Input: part model. Units: mm. Frame: model coordinates. A direction names the side the tool comes from. Coordinates: 2 decimals unless noted, no trailing zeros. Write each loop counter-clockwise with the first axis right and the second up, starting at its lowest first coordinate (ties: lowest second). Pieces come first, ordered by that corner, then holes. Notation, with made-up numbers: (52, 28) - (71, 28) arc R17 ccw to (71, 35) - close; hole circle Ø3 at (70, 41.25). An arc over 180 degrees is marked (long way). Put each result on its own line as item: value. Start each with the question number.
1. Cut plane C-C, the plane y = 31.5. Return loops of the section in (x, z), and give its area (3 significant figures).
2. Pull-direction query (X, two-part tool) for faces 1 (the flat face through (1, 10, -42)), 2 (the flat face through (60, 10, 0)), 3 (the flat face through (-32, 10, -37)), 4 (the cylindrical face through (-60.859, 21.256, -40.797)); classes: released by +X, released by -X, zero draft, split by the parting line, or undercut.
3. Line query: line 1 (Z direction, x = 47, y = 7); line 2 (X direction, y = 10.5, z = 24.5); line 3 (Z direction, x = -31, y = 17). Output: solid intervals per line, ascending.
4. Access query for faces 5 (the flat face through (62, 9, -1)), 6 (the flat face through (10, 10, 40)). Directions: +Z, -Z, +X, -X, +Y, -Y. A direction counts if a zero-diameter tool reaches every point of the face in a straight line with its end or side. Return the directions, or none.
5. Pin query (flat end, axial travel): pin 1 (1.8 mm diameter, centred on y = 25, z = 35.5, fed in from +X); pin 2 (12 mm diameter, centred on x = -34, z = -13, fed in from +Y); pin 3 (1.5 mm diameter, centred on y = 34, z = 33, fed in from +X). Return the tip coordinate at first contact, or that it passes through.
6. Cut plane D-D, the plane y = 40. Return loops of the section in (x, z), and give its area (3 significant figures).
7. Cut plane B-B, the plane z = 20.5. Return loops of the section in (x, y), and give its area (3 significant figures).
8. Cut plane A-A, the plane x = 30.5. Return loops of the section in (y, z), and give its area (3 significant figures).
from build123d import *

# Parameters (mm, degrees)
SKETCH1_W            = 124
SKETCH1_H            = 84
SKETCH1_W_2          = 120
SKETCH1_H_2          = 80
EXTRUDE_THIN1_DEPTH  = 20
SKETCH2_W            = 124
SKETCH2_H            = 84
BOSS_EXTRUDE1_DEPTH  = 2
BOSS_EXTRUDE2_DEPTH  = 6
SKETCH9_W            = 6
SKETCH9_H            = 6
BOSS_EXTRUDE7_DEPTH  = 20
BOSS_EXTRUDE8_DEPTH  = 2
BOSS_EXTRUDE9_START  = -2
BOSS_EXTRUDE9_DEPTH  = 6
BOSS_EXTRUDE10_DEPTH = 68
FILLET1_R            = 4


with BuildPart() as part:
    # Sketch1 → Extrude-Thin1 (new body)
    with BuildSketch(Plane(origin=(0, 0, 0), x_dir=(1, 0, 0), z_dir=(0, 1, 0))):
        Rectangle(SKETCH1_W, SKETCH1_H)
        Rectangle(SKETCH1_W_2, SKETCH1_H_2, mode=Mode.SUBTRACT)
    extrude(amount=EXTRUDE_THIN1_DEPTH)

    # Sketch2 → Boss-Extrude1 (add)
    with BuildSketch(Plane.XZ):
        Rectangle(SKETCH2_W, SKETCH2_H)
    extrude(amount=BOSS_EXTRUDE1_DEPTH)

    # Sketch3 → Boss-Extrude2 (add)
    with BuildSketch(Plane.XY.offset(-40)):
        Polygon((-24, 13.287202951), (-24, -2), (-32, -2), (-32, 20), align=None)
    boss_extrude2 = extrude(amount=BOSS_EXTRUDE2_DEPTH)

    # Sketch9 → Boss-Extrude7 (add)
    with BuildSketch(Plane(origin=(0, 20, 0), x_dir=(1, 0, 0), z_dir=(0, 1, 0))):
        with Locations((57, 37)):
            Rectangle(SKETCH9_W, SKETCH9_H)
        with Locations((57, -37)):
            Rectangle(SKETCH9_W, SKETCH9_H)
    extrude(amount=-BOSS_EXTRUDE7_DEPTH)

    # Sketch10 → Boss-Extrude8 (add)
    with BuildSketch(Plane(origin=(0, 0, -42), x_dir=(-1, 0, 0), z_dir=(0, 0, -1))):
        Polygon((62, 20), (62, 45.172988935), (32, 20), align=None)
    boss_extrude8 = extrude(amount=-BOSS_EXTRUDE8_DEPTH)

    # Sketch11 → Boss-Extrude9 (add)
    with BuildSketch(Plane(origin=(0, 0, -42), x_dir=(-1, 0, 0), z_dir=(0, 0, -1)).offset(BOSS_EXTRUDE9_START)):
        Polygon((62, 45.172988935), (49.619022192, 34.784115023), (49.619022192, -2), (62, -2), align=None)
    boss_extrude9 = extrude(amount=-BOSS_EXTRUDE9_DEPTH)

    # Mirror1: Boss-Extrude2, Boss-Extrude8, Boss-Extrude9 across plane
    add(boss_extrude2.mirror(Plane(origin=(0, 0, 0), x_dir=(1, 0, 0), z_dir=(0, 0, -1))))
    add(boss_extrude8.mirror(Plane(origin=(0, 0, 0), x_dir=(1, 0, 0), z_dir=(0, 0, -1))))
    add(boss_extrude9.mirror(Plane(origin=(0, 0, 0), x_dir=(1, 0, 0), z_dir=(0, 0, -1))))

    # Sketch12 → Boss-Extrude10 (add)
    with BuildSketch(Plane.XY.offset(-34)):
        Polygon((-62, 20), (-62, 45.172988935), (-60, 43.494789673), (-60, 20), align=None)
    extrude(amount=BOSS_EXTRUDE10_DEPTH)

    # Fillet1
    fillet1_edges = [part.edges().sort_by_distance(p)[0] for p in [
        (62, 9, 42),
        (-62, 21.586494468, 42),
        (-62, 21.586494468, -42),
        (62, 9, -42),
        (54, 10, -34),
        (54, 10, 34),
    ]]
    fillet(fillet1_edges, radius=FILLET1_R)


solid = part.part
Report:
1. outline: (-62, -38) arc R4 ccw to (-58, -42) - (-45.71, -42) - (-45.71, -40) - (-49.62, -40) - (-49.62, -34) - (-60, -34) - (-60, 34) - (-49.62, 34) - (-49.62, 40) - (-45.71, 40) - (-45.71, 42) - (-58, 42) arc R4 ccw to (-62, 38) - close
1. area: 343 mm^2
2. face 1: zero draft
2. face 2: undercut
2. face 3: undercut
2. face 4: released by -X
3. line 1: z = -42 to -40, 40 to 42
3. line 2: x = -62 to -60, 60 to 62
3. line 3: z = -42 to -34, 34 to 42
4. face 5: +Z, -Z, +X, +Y, -Y
4. face 6: +Y
5. pin 1: stops at x = -49.62
5. pin 2: stops at y = 0
5. pin 3: stops at x = -60
6. outline: (-62, -38) arc R4 ccw to (-58, -42) - (-55.84, -42) - (-55.84, -34) - (-60, -34) - (-60, 34) - (-55.84, 34) - (-55.84, 42) - (-58, 42) arc R4 ccw to (-62, 38) - close
6. area: 228 mm^2
7. outline: (-62, -2) - (62, -2) - (62, 20) - (60, 20) - (60, 0) - (-60, 0) - (-60, 43.49) - (-62, 45.17) - close
7. area: 377 mm^2
8. outline: (-2, -42) - (20, -42) - (20, -40) - (0, -40) - (0, 40) - (20, 40) - (20, 42) - (-2, 42) - close
8. area: 248 mm^2
